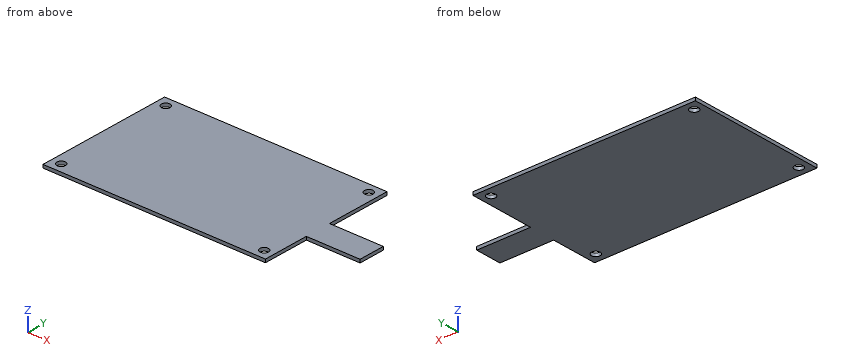
from build123d import *

# Parameters (mm, degrees)
SKETCH_R  = 1
PAD_DEPTH = 0.75


with BuildPart() as part:
    # Sketch → Pad (new body)
    with BuildSketch(Plane.XY):
        Polygon((-25.85, 16.125), (25.85, 16.125), (25.85, 0.875), (38.35, 0.875), (38.35, -5.275), (25.85, -5.275), (25.85, -16.125), (-25.85, -16.125), align=None)
        with Locations((-23.6, 13.875)):
            Circle(SKETCH_R, mode=Mode.SUBTRACT)
        with Locations((23.6, -13.875)):
            Circle(SKETCH_R, mode=Mode.SUBTRACT)
        with Locations((23.6, 13.875)):
            Circle(SKETCH_R, mode=Mode.SUBTRACT)
        with Locations((-23.6, -13.875)):
            Circle(SKETCH_R, mode=Mode.SUBTRACT)
    extrude(amount=PAD_DEPTH)


solid = part.part
Here's how the part is built. I have some questions about the finished solid (model axes, mm). Round coordinates to 2 decimals unless told otherwise and drop trailing zeros. Loops run counter-clockwise (first coordinate to the right, second up) from the corner with the lowest first, then second, coordinate; pieces in that order, holes last.
1. If I drill on line 1 along X through (y, z) = (14, 0.15); line 2 along Y through (x, z) = (-23.6, 0.6) (3 decimals); line 3 along X through (y, z) = (-9, 0.05), over which ranges is the centre line in solid material (lowest first)?
Answer list:
line 1: x = -25.85 to -24.59, -22.61 to 22.61, 24.59 to 25.85
line 2: y = -16.125 to -14.875, -12.875 to 12.875, 14.875 to 16.125
line 3: x = -25.85 to 25.85
2. If we section it at B-B on z = 0.6: Write out the boundary of the cut face in (x, y) (3 decimals), plus the area to 3 significant figures.
Answer list:
outline: (-25.85, -16.125) - (25.85, -16.125) - (25.85, -5.275) - (38.35, -5.275) - (38.35, 0.875) - (25.85, 0.875) - (25.85, 16.125) - (-25.85, 16.125) - close; hole circle Ø2 at (-23.6, -13.875); hole circle Ø2 at (-23.6, 13.875); hole circle Ø2 at (23.6, -13.875); hole circle Ø2 at (23.6, 13.875)
area: 1,730 mm2
3. If we section it at A-A on x = -23.6: Write out the boundary of the cut face in (y, z) (3 decimals), plus the area to 3 significant figures.
Answer list:
outline: (-16.125, 0) - (-14.875, 0) - (-14.875, 0.75) - (-16.125, 0.75) - close; (-12.875, 0) - (12.875, 0) - (12.875, 0.75) - (-12.875, 0.75) - close; (14.875, 0) - (16.125, 0) - (16.125, 0.75) - (14.875, 0.75) - close
area: 21.2 mm2
4. If we section it at C-C on y = 12: Write out the boundary of the cut face in (x, z), plus the area to 3 significant figures.
Answer list:
outline: (-25.85, 0) - (25.85, 0) - (25.85, 0.75) - (-25.85, 0.75) - close
area: 38.8 mm2
5. For P1, Ø3, axis at x = 23.6, y = 13.875, coming from the +Z side, with a flat end and sliding along its axis, tell me the tip position at first contact or that it passes through.
Answer list:
P1: stops at z = 0.75
6. If we section it at D-D on x = 29: Write out the boundary of the cut face in (y, z) (3 decimals).
Answer list:
outline: (-5.275, 0) - (0.875, 0) - (0.875, 0.75) - (-5.275, 0.75) - close
